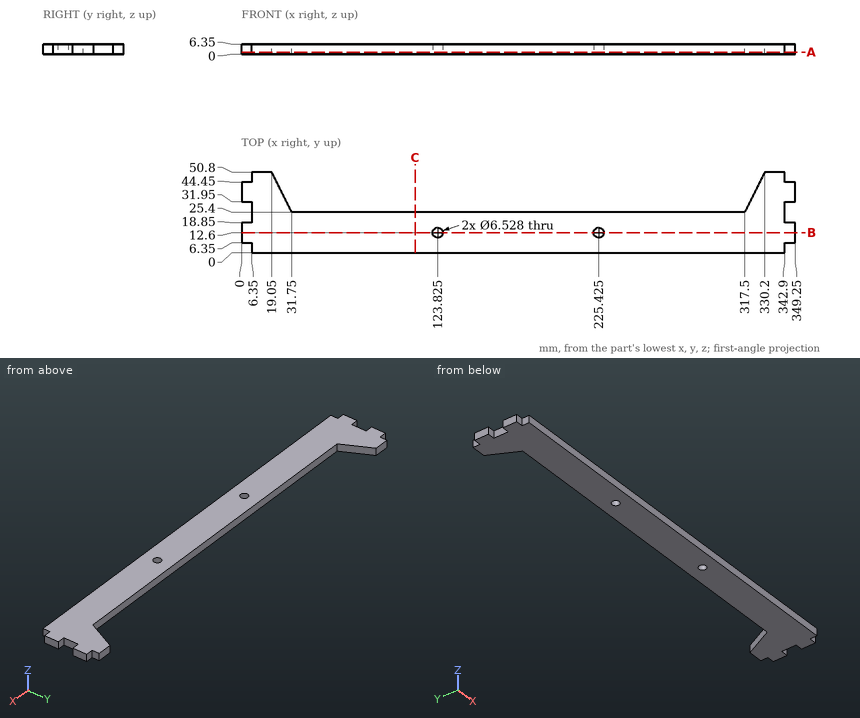
Geometry check sheet. Reference: drawing and pictorial views, mm from the part's lowest x, y, z. Give positions to 0.01 mm unless a question says otherwise; leave off trailing zeros. Write each loop counter-clockwise with the first axis right and the second up, starting at its lowest first coordinate (ties: lowest second). Pieces come first, ordered by that corner, then holes. Notation, with made-up numbers: (41.25, 22.5) -> (55.25, 22.5) arc R23 cw to (55.25, 45.5) -> close; hole circle Ø7 at (47.5, 60.5). An arc over 180 degrees is marked (long way). One line per question, with ' | ' between items.
Item 1: Scan lines: line 1 along X through (y, z) = (14, 1.25); line 2 along Y through (x, z) = (44, 2.5); line 3 along X through (y, z) = (4.5, 4). Record each from-to range of solid material in increasing order.
Determined:
line 1: 0 to 120.88, 126.77 to 222.48, 228.37 to 349.25 | line 2: 0 to 25.4 | line 3: 6.35 to 342.9
Item 2: Sectioned sample at B-B, the plane y = 12.6. Record the boundary of the cut face in (x, z).
Determined:
outline: (0, 0) -> (120.56, 0) -> (120.56, 6.35) -> (0, 6.35) -> close; (127.09, 0) -> (222.16, 0) -> (222.16, 6.35) -> (127.09, 6.35) -> close; (228.69, 0) -> (349.25, 0) -> (349.25, 6.35) -> (228.69, 6.35) -> close
Item 3: Depth check by flat-ended pin: pin 1 (3 mm diameter, centred on x = 345, z = 2.5, fed in from -Y); pin 2 (1.9 mm diameter, centred on y = 28, z = 2.5, fed in from +X); pin 3 (1.5 mm diameter, centred on x = 172.5, z = 4.5, fed in from +Y); pin 4 (5 mm diameter, centred on x = 225.425, y = 12.6, fed in from +Z). Enter the tip coordinate at first touch or a pass-through.
Determined:
pin 1: y = 6.35 | pin 2: x = 342.9 | pin 3: y = 25.4 | pin 4: through
Item 4: Sectioned sample at C-C, the plane x = 109.5. Record the boundary of the cut face in (y, z), plus the area to 3 significant figures.
Determined:
outline: (0, 0) -> (25.4, 0) -> (25.4, 6.35) -> (0, 6.35) -> close | area: 161 mm^2
Item 5: Sectioned sample at A-A, the plane z = 1.25. State how many separate pieces and enclosed holes the cut face has, plus the area to 3 significant figures.
Determined:
separate pieces: 1 | enclosed holes: 2 | area: 9,770 mm^2
